Here's how the part is built. I have some questions about the finished solid (model axes, mm). A direction names the side the tool comes from. Round coordinates to 2 decimals unless told otherwise and drop trailing zeros. Write each loop counter-clockwise with the first axis right and the second up, starting at its lowest first coordinate (ties: lowest second). Pieces come first, ordered by that corner, then holes. Notation, with made-up numbers: (19.5, -17.75) -> (41.5, -17.75) arc R28 cw to (41.5, 5.25) -> close; hole circle Ø3 at (-20, -19.75). An arc over 180 degrees is marked (long way). Answer in a Markdown table with one row per item.
Autodesk Inventor part; units mm, degrees
ref_plane "YZ Plane" through (0, 0, 0) normal (1, 0, 0) x (0, 1, 0)
ref_plane "XZ Plane" through (0, 0, 0) normal (0, 1, 0) x (-1, 0, 0)
ref_plane "XY Plane" through (0, 0, 0) normal (0, 0, 1) x (1, 0, 0)
sketch "Sketch1" plane through (0, 0, 0) normal (0, 0, 1) x (1, 0, 0)
  line L0 (0, 0) -> (0, 76.2)
  line L1 (0, 76.2) -> (-25.4, 76.2)
  line L2 (-25.4, 76.2) -> (-25.4, 635)
  line L3 (-25.4, 635) -> (3.175, 635)
  line L4 (3.175, 635) -> (3.175, 685.8)
  line L5 (3.175, 685.8) -> (377.825, 685.8)
  line L6 (377.825, 685.8) -> (377.825, 635)
  line L7 (377.825, 635) -> (406.4, 635)
  line L8 (406.4, 635) -> (406.4, 76.2)
  line L9 (406.4, 76.2) -> (381, 76.2)
  line L10 (381, 76.2) -> (381, 0)
  line L11 (381, 0) -> (0, 0)
  dimension "d0" = 76.2
  dimension "d1" = 25.4
  dimension "d2" = 558.8
  dimension "d3" = 28.575
  dimension "d4" = 50.8
  dimension "d5" = 374.65
  dimension "d6" = 28.575
  dimension "d7" = 25.4
extrude "Extrusion1" add sketch "Sketch1" along normal blind 19.05
sketch "Sketch2" plane through (0, 0, 19.05) normal (0, 0, 1) x (1, 0, 0)
  point P0 (0, 0)
sketch "Sketch3" plane through (0, 0, 19.05) normal (0, 0, 1) x (1, 0, 0)
  line L0 (-25.4, 635) -> (-25.4, 76.2) construction
  line L1 (-25.4, 635) -> (-25.4, 369.062) construction
  line L2 (-25.4, 369.062) -> (-16.9333, 369.062) construction
  line L3 (-25.4, 369.062) -> (-16.9333, 369.062) construction
  line L4 (-16.9333, 369.062) -> (84.6667, 369.062) construction
  line L5 (-25.4, 76.2) -> (-25.4, 306.324) construction
  line L6 (-25.4, 306.324) -> (-16.9333, 306.324) construction
  line L7 (-16.9333, 306.324) -> (84.6667, 306.324) construction
  circle A0 centre (84.6667, 369.062) radius 2.5797
  circle A1 centre (-16.9333, 369.062) radius 2.5797
  circle A2 centre (84.6667, 306.324) radius 2.5797
  circle A3 centre (-16.9333, 306.324) radius 2.5797
  line L8 (377.825, 685.8) -> (3.175, 685.8) construction
  line L9 (190.5, 685.8) -> (190.5, 0) construction
  line L10 (0, 0) -> (381, 0) construction
  line L11 (190.5, 0) -> (165.1, 0) construction
  line L12 (165.1, 0) -> (165.1, 12.7) construction
  circle A4 centre (165.1, 12.7) radius 2.5797
  line L13 (190.5, 685.8) -> (165.1, 685.8) construction
  line L14 (165.1, 685.8) -> (165.1, 673.1) construction
  circle A5 centre (165.1, 673.1) radius 2.5797
  line L15 (406.4, 635) -> (406.4, 76.2) construction
  line L16 (406.4, 635) -> (406.4, 369.062) construction
  line L17 (406.4, 76.2) -> (406.4, 306.324) construction
  line L18 (3.175, 685.8) -> (377.825, 685.8) construction
  line L19 (381, 0) -> (0, 0) construction
  line L20 (190.5, 0) -> (215.9, 0) construction
  line L21 (215.9, 0) -> (215.9, 12.7) construction
  circle A6 centre (215.9, 12.7) radius 2.5797
  line L22 (190.5, 685.8) -> (215.9, 685.8) construction
  line L23 (215.9, 685.8) -> (215.9, 673.1) construction
  circle A7 centre (215.9, 673.1) radius 2.5797
  line L24 (406.4, 76.2) -> (406.4, 635)
  line L25 (406.4, 685.8) -> (406.4, 382.5189) construction
  line L26 (406.4, 382.5189) -> (395.1148, 382.5189) construction
  line L27 (395.1148, 382.5189) -> (293.5148, 382.5189) construction
  line L28 (293.5148, 382.5189) -> (293.5148, 319.7809) construction
  line L29 (293.5148, 319.7809) -> (395.1148, 319.7809) construction
  circle A8 centre (395.1148, 382.5189) radius 2.5797
  circle A9 centre (293.5148, 382.5189) radius 2.5797
  circle A10 centre (293.5148, 319.7809) radius 2.5797
  circle A11 centre (395.1148, 319.7809) radius 2.5797
  dimension "d10" = 265.938
  dimension "d11" = 8.4667
  dimension "d12" = 0
  dimension "d13" = 101.6
  dimension "d14" = 230.124
  dimension "d15" = 5.1594
  dimension "d16" = 25.4
  dimension "d17" = 12.7
  dimension "d19" = 5.1594
  dimension "d20" = 25.4
  dimension "d21" = 12.7
  dimension "d25" = 303.2811
  dimension "d26" = 11.2852
  dimension "d27" = 101.6
  dimension "d28" = 62.738
  dimension "d29" = 5.1594
extrude "Extrusion2" cut sketch "Sketch3" against normal blind 25.4
properties part number "Arm Belly Pan"
1) For pin 1 (5.5 mm diameter, centred on x = -17, z = 6.5, fed in from -Y); pin 2 (4.5 mm diameter, centred on x = 215.9, y = 673.1, fed in from +Z); pin 3 (9.5 mm diameter, centred on y = 666, z = 7.5, fed in from +X) (3 decimals), each with a flat end and sliding along its axis, tell me the tip position at first contact or that it passes through.
Response:
| item | result |
|---|---|
| pin 1 | stops at y = 76.2 |
| pin 2 | passes through |
| pin 3 | stops at x = 377.825 |
2) I need wall thicknesses on line 1 (Y direction, x = 165.1, z = 9); line 2 (X direction, y = 641.5, z = 18) (3 decimals); line 3 (X direction, y = 60, z = 7.75). Which ranges of each line are inside material? Lowest first, please. Write a range as [from, to].
Response:
| item | result |
|---|---|
| line 1 | y = [0, 10.12], [15.28, 670.52], [675.68, 685.8] |
| line 2 | x = [3.175, 377.825] |
| line 3 | x = [0, 381] |
3) I want a section at A-A, the plane z = 7.25. Count the separate pieces of the cut face and the enclosed holes in it, and give its area (3 significant figures).
Response:
| item | result |
|---|---|
| separate pieces | 1 |
| enclosed holes | 12 |
| area | 289,000 mm^2 |
4) Which directions (+Z, -Z, +X, -X, +Y, -Y) give clear straight access to the entire face, cutting with the end or side of a thin tool? Please do faces 1 (the face through (-11, 635, 9)), 2 (the face through (392, 635, 9)), 3 (the face through (381, 39, 9)).
Response:
| item | result |
|---|---|
| face 1 | +Z, -Z, -X, +Y |
| face 2 | +Z, -Z, +X, +Y |
| face 3 | +Z, -Z, +X, -Y |
5) I want a section at B-B, the plane y = 56. List the corners of the cut face in (x, z) for me, and give its area (3 significant figures).
Response:
| item | result |
|---|---|
| outline | (0, 0) -> (381, 0) -> (381, 19.05) -> (0, 19.05) -> close |
| area | 7,260 mm^2 |
